from build123d import *

# Parameters (mm, degrees)
SKETCH1_R                     = 1.5
BOSS_EXTRUDE1_DEPTH           = 7.5
BOSS_EXTRUDE3_DEPTH           = 5
BOSS_EXTRUDE3_DRAFT           = 10
BOSS_EXTRUDE3_PROFILE_2_DEPTH = 5
BOSS_EXTRUDE3_PROFILE_2_DRAFT = 10


with BuildPart() as part:
    # Sketch1 → Boss-Extrude1 (new body)
    with BuildSketch(Plane.XY):
        with BuildLine():
            Line((2.549509757, 2.75), (32.549509757, 2.75))
            Line((32.549509757, 2.75), (32.549509757, -2.75))
            Line((32.549509757, -2.75), (22.049509757, -2.75))
            Line((22.049509757, -2.75), (2.549509757, -2.75))
            ThreePointArc((2.549509757, -2.75), (-3.75, 0), (2.549509757, 2.75))
        make_face()
        Circle(SKETCH1_R, mode=Mode.SUBTRACT)
    extrude(amount=BOSS_EXTRUDE1_DEPTH)


with BuildPart() as boss_extrude3_tool:
    # Sketch2 → Boss-Extrude3 (with draft: the straight prism first)
    with BuildSketch(Plane.XZ.offset(2.75)):
        with BuildLine():
            Line((31.973749775, 7.5), (27.204053767, 6))
            ThreePointArc((27.204053767, 6), (27.549509757, 3.75), (27.204053767, 1.5))
            Line((27.204053767, 1.5), (31.973749775, 0))
            ThreePointArc((31.973749775, 0), (32.549509757, 3.75), (31.973749775, 7.5))
        make_face()
    extrude(amount=BOSS_EXTRUDE3_DEPTH)
    # Boss-Extrude3: the draft: its side faces are tilted about the plane it starts from
    boss_extrude3_sides = [boss_extrude3_tool.faces().sort_by_distance(p)[0] for p in [
        (32.549509757, -5.25, 3.75),
        (29.588901771, -5.25, 6.75),
        (27.549509757, -5.25, 3.75),
        (29.588901771, -5.25, 0.75),
    ]]
    draft(boss_extrude3_sides, Plane.XZ.offset(2.75), BOSS_EXTRUDE3_DRAFT)


with BuildPart() as part_1:
    add(part.part)

    # Boss-Extrude3: add boss_extrude3_tool
    add(boss_extrude3_tool.part)


with BuildPart() as boss_extrude3_profile_2_tool:
    # Sketch2 → Boss-Extrude3 profile 2 (with draft: the straight prism first)
    with BuildSketch(Plane.XZ.offset(2.75)):
        with BuildLine():
            ThreePointArc((8.125269739, 7.5), (7.549509757, 3.75), (8.125269739, 0))
            Line((8.125269739, 0), (12.894965746, 1.5))
            ThreePointArc((12.894965746, 1.5), (12.549509757, 3.75), (12.894965746, 6))
            Line((12.894965746, 6), (8.125269739, 7.5))
        make_face()
    extrude(amount=BOSS_EXTRUDE3_PROFILE_2_DEPTH)
    # Boss-Extrude3 profile 2: the draft: its side faces are tilted about the plane it starts from
    boss_extrude3_profile_2_sides = [boss_extrude3_profile_2_tool.faces().sort_by_distance(p)[0] for p in [
        (10.510117743, -5.25, 0.75),
        (12.549509757, -5.25, 3.75),
        (10.510117743, -5.25, 6.75),
        (7.549509757, -5.25, 3.75),
    ]]
    draft(boss_extrude3_profile_2_sides, Plane.XZ.offset(2.75), BOSS_EXTRUDE3_PROFILE_2_DRAFT)


with BuildPart() as part_2:
    add(part_1.part)

    # Boss-Extrude3 profile 2: add boss_extrude3_profile_2_tool
    add(boss_extrude3_profile_2_tool.part)


solid = part_2.part
The model under review builds one solid part; all positions refer to its coordinate system, in mm. A direction names the side the tool comes from. Coordinates: 2 decimals unless noted, no trailing zeros. Write each loop counter-clockwise with the first axis right and the second up, starting at its lowest first coordinate (ties: lowest second). Pieces come first, ordered by that corner, then holes. Notation, with made-up numbers: M -19,68 L 23,68 A21 ccw 23,93 Z; hole C -24.5,66.25 d11. An arc over 180 degrees is marked long. Put each result on its own line as item: value.
1) Draft analysis for pull direction Z (two halves, no side actions). For faces 1 (the conical face through (12.115, -5.215, 3.716)), 2 (the flat face through (32.55, 0, 4)), 3 (the flat face through (15, 0, 7.5)), state which applies: released by +Z, released by -Z, zero draft, split by the parting line, or undercut.
Computed:
face 1: undercut
face 2: zero draft
face 3: released by +Z
2) Wall thickness on probe 1 along X at (y, z) = (-3, 5.75); probe 2 along Y at (x, z) = (0, 4.75); probe 3 along Y at (x, z) = (15.5, 1.75): over which ranges is each line inside the solid? List them lowest first. Write a range as [from, to].
Computed:
probe 1: x = [-2.25, 2.25], [7.76, 12.78], [27.32, 32.34]
probe 2: y = [-3.75, -1.5], [1.5, 3.75]
probe 3: y = [-2.75, 2.75]
3) Clearance check with flat-ended pins moving along their axes: pin 1 Ø1.5 at (y, z) = (-0.5, 2) entering from -X; pin 2 Ø4 at (x, z) = (18.5, 4.5) entering from +Y; pin 3 Ø1.5 at (y, z) = (-3, 6) entering from -X; pin 4 Ø2 at (x, z) = (16, 3.5) entering from -Y. State where each tip first meets the part, or that it passes through.
Computed:
pin 1: stops at x = -3.75
pin 2: stops at y = 2.75
pin 3: stops at x = -3
pin 4: stops at y = -2.75
4) Add section D-D on x = 23.5. Give the boundary of the cut face in (y, z).
Computed:
outline: M -2.75,0 L 2.75,0 L 2.75,7.5 L -2.75,7.5 Z
5) For faces 4 (the flat face through (10, -7.75, 4)), 5 (the flat face through (17, 2.75, 4)), 6 (the conical face through (27.984, -5.215, 3.784)), 7 (the flat face through (10.413, -5.215, 6.325)), 8 (the flat face through (29.686, -5.215, 1.175)), list the 3-axis set-ups (+Z, -Z, +X, -X, +Y, -Y) from which the entire face can be reached by the end or side of a thin tool; tool diameter is ignored.
Computed:
face 4: +Z, -Z, +X, -X, -Y
face 5: +Z, -Z, +X, +Y
face 6: -Y
face 7: +Z, -Y
face 8: -Z, -Y
6) Add section B-B on x = 0. Give the boundary of the cut face in (y, z).
Computed:
outline: M -3.75,0 L -1.5,0 L -1.5,7.5 L -3.75,7.5 Z; M 1.5,0 L 3.75,0 L 3.75,7.5 L 1.5,7.5 Z
7) Add section A-A on y = 0. Give the boundary of the cut face in (x, z), then the cut area to 3 significant figures.
Computed:
outline: M -3.75,0 L -1.5,0 L -1.5,7.5 L -3.75,7.5 Z; M 1.5,0 L 32.55,0 L 32.55,7.5 L 1.5,7.5 Z
area: 250 mm2
8) Add section C-C on x = 29. Give the boundary of the cut face in (y, z).
Computed:
outline: M -7.75,1.86 L -2.75,0.94 L -2.75,0 L 2.75,0 L 2.75,7.5 L -2.75,7.5 L -2.75,6.56 L -7.75,5.64 Z
